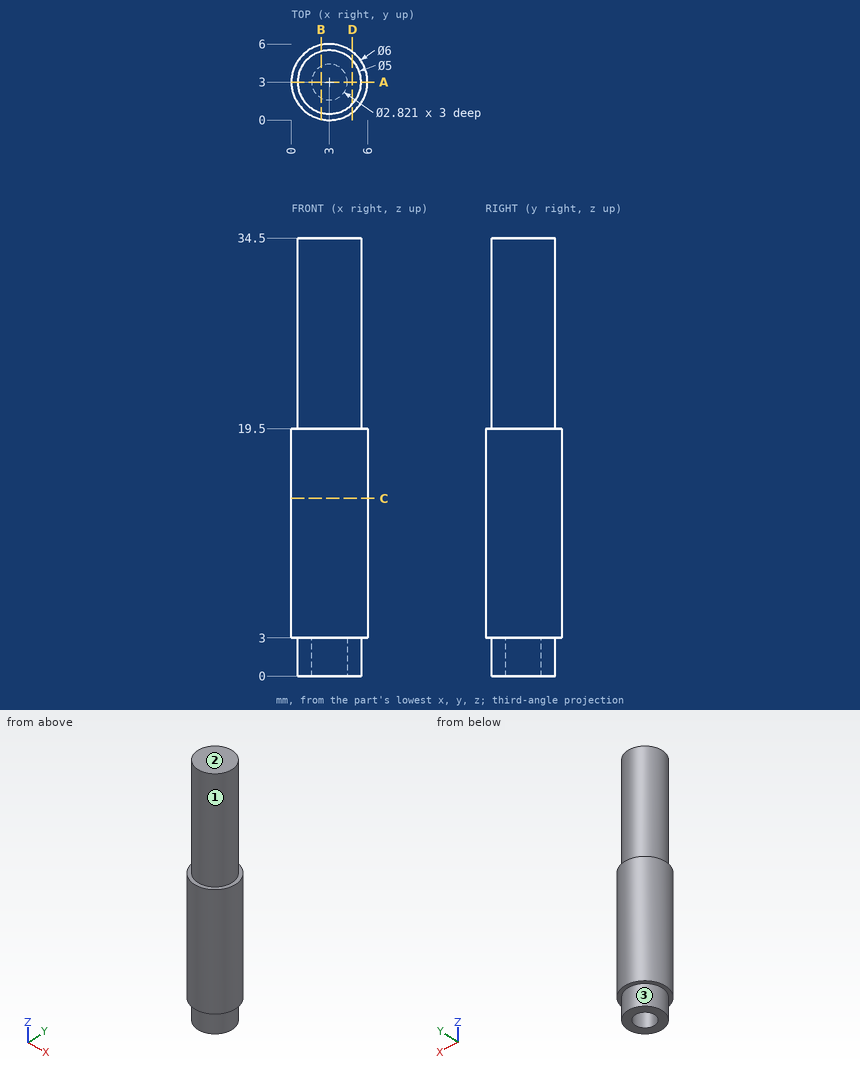
Geometry check sheet. Reference: drawing and pictorial views, mm from the part's lowest x, y, z. A direction names the side the tool comes from. Round coordinates to 2 decimals unless told otherwise and drop trailing zeros. Loops run counter-clockwise (first coordinate to the right, second up) from the corner with the lowest first, then second, coordinate; pieces in that order, holes last. Notation, with made-up numbers: (68, -4.75) - (126, -4.75) arc R27 cw to (126, 29.25) - close; hole circle Ø7 at (55.5, 31). An arc over 180 degrees is marked (long way). One line per question, with ' | ' between items. Start each with the question number.
1. Cross-section at B-B on x = 2.35. Record the cut outline in (y, z), then the cut area to 3 significant figures.
2. Scan lines: line 1 (Y direction, x = 3, z = 0.6); line 2 (Z direction, x = 4.6, y = 5.05); line 3 (Z direction, x = 2.35, y = 4.1). Record each from-to range of solid material in increasing order. Write a range as [from, to].
3. Cross-section at C-C on z = 14. Record the cut outline in (x, y), then the cut area to 3 significant figures.
4. Depth check by flat-ended pin: pin 1 (3 mm diameter, centred on x = 3, z = 26.5, fed in from +Y); pin 2 (1 mm diameter, centred on y = 4.5, z = 17.5, fed in from +X); pin 3 (0.8 mm diameter, centred on x = 3, y = 3, fed in from -Z). Enter the tip coordinate at first touch or a pass-through.
5. Cross-section at A-A on y = 3. Record the cut outline in (x, z).
6. Tool access check on the marked faces 1, 2 and 3. Record the directions out of +Z, -Z, +X, -X, +Y, -Y that give a thin tool (end or side, any length) a straight path to the whole face; none if there is none.
7. Cross-section at D-D on x = 4.8. Record the cut outline in (y, z) (1 decimal).
Taken from the geometry:
1) outline: (0.07, 3) - (0.59, 3) - (0.59, 0) - (1.75, 0) - (1.75, 3) - (4.25, 3) - (4.25, 0) - (5.41, 0) - (5.41, 3) - (5.93, 3) - (5.93, 19.5) - (5.41, 19.5) - (5.41, 34.5) - (0.59, 34.5) - (0.59, 19.5) - (0.07, 19.5) - close | area: 176 mm²
2) line 1: [0.5, 1.59], [4.41, 5.5] | line 2: [3, 19.5] | line 3: [3, 34.5]
3) outline: circle Ø6 at (3, 3) | area: 28.3 mm²
4) pin 1: y = 5.5 | pin 2: x = 5.83 | pin 3: z = 3
5) outline: (0, 3) - (0.5, 3) - (0.5, 0) - (1.59, 0) - (1.59, 3) - (4.41, 3) - (4.41, 0) - (5.5, 0) - (5.5, 3) - (6, 3) - (6, 19.5) - (5.5, 19.5) - (5.5, 34.5) - (0.5, 34.5) - (0.5, 19.5) - (0, 19.5) - close
6) face 1: +Z | face 2: +Z, +X, -X, +Y, -Y | face 3: -Z
7) outline: (0.6, 3) - (1.3, 3) - (1.3, 0) - (4.7, 0) - (4.7, 3) - (5.4, 3) - (5.4, 19.5) - (4.7, 19.5) - (4.7, 34.5) - (1.3, 34.5) - (1.3, 19.5) - (0.6, 19.5) - close
